Build history of the part. All positions in model axes, mm. A direction names the side the tool comes from. Round coordinates to 2 decimals unless told otherwise and drop trailing zeros. Write each loop counter-clockwise with the first axis right and the second up, starting at its lowest first coordinate (ties: lowest second). Pieces come first, ordered by that corner, then holes. Notation, with made-up numbers: M 47,87 L 57,87 A24 cw 57,115 Z; hole C 84,26 d9. An arc over 180 degrees is marked long. One line per item, written item: value. Start each with the question number.
```python
from build123d import *

# Parameters (mm, degrees)
F0_R     = 2.38125
F1_DEPTH = 3.175
F2_DEPTH = 4.7625
F3_T     = -1.5875
F4_R     = 3.175
F4_R_2   = 2.38125
F5_DEPTH = 1.5875


with BuildPart() as f1:
    # F0 (on Top) → F1 (new body)
    with BuildSketch(Plane.XY):
        Polygon((0, 15.875), (-7.9375, 15.875), (-7.9375, -15.875), (7.9375, -15.875), align=None)
        with Locations((-3.96875, -11.90625)):
            Circle(F0_R, mode=Mode.SUBTRACT)
        with Locations((-3.96875, -3.96875)):
            Circle(F0_R, mode=Mode.SUBTRACT)
        with Locations((-3.96875, 3.96875)):
            Circle(F0_R, mode=Mode.SUBTRACT)
        with Locations((-3.96875, 11.90625)):
            Circle(F0_R, mode=Mode.SUBTRACT)
    extrude(amount=F1_DEPTH)

    # F0 (on Top) → F2 (join)
    with BuildSketch(Plane.XY):
        with Locations((-3.96875, 11.90625)):
            Circle(F0_R)
        with Locations((-3.96875, 3.96875)):
            Circle(F0_R)
        with Locations((-3.96875, -3.96875)):
            Circle(F0_R)
        with Locations((-3.96875, -11.90625)):
            Circle(F0_R)
    extrude(amount=F2_DEPTH)

    # F3
    f3_openings = [f1.faces().sort_by_distance(p)[0] for p in [
        (-1.763889, -1.763889, 0),
    ]]
    offset(amount=F3_T, openings=f3_openings, kind=Kind.INTERSECTION)

    # F2_face (on face) + F4 (on face) → F5 (join)
    with BuildSketch(Plane(origin=(-1.7638745265, -1.3908157983, 0), x_dir=(1, 0, 0), z_dir=(0, 0, -1))):
        Polygon((-6.1736254735, -17.2658157983), (1.7638745265, -17.2658157983), (9.7013745265, 14.4841842017), (-6.1736254735, 14.4841842017), align=None)
        Polygon((0.5243919814, -15.6783157983), (-4.5861254735, -15.6783157983), (-4.5861254735, 12.8966842017), (7.6681419814, 12.8966842017), align=None, mode=Mode.SUBTRACT)
    with BuildSketch(Plane(origin=(0, 0, 1.5875), x_dir=(1, 0, 0), z_dir=(0, 0, -1))):
        with BuildLine():
            Line((0.8992491716, -5.7325731328), (1.0932302062, -4.9566489946))
            ThreePointArc((1.0932302062, -4.9566489946), (-3.080202438, -7.1674493905), (-0.4381385265, -11.0821239253))
            Line((-0.4381385265, -11.0821239253), (-0.244157492, -10.3061997871))
            ThreePointArc((-0.244157492, -10.3061997871), (-2.3101518285, -7.3599620429), (0.8992491716, -5.7325731328))
        make_face()
        with BuildLine():
            ThreePointArc((2.7353766172, 1.6119366495), (-3.080202438, 0.7700506095), (1.6550091801, -2.7095330988))
            Line((1.6550091801, -2.7095330988), (2.0152745824, -1.2684714896))
            ThreePointArc((2.0152745824, -1.2684714896), (-2.3101518285, 0.5775379571), (2.3751112149, 0.1708750402))
            Line((2.3751112149, 0.1708750402), (2.7353766172, 1.6119366495))
        make_face()
        with Locations((0, 7.9375)):
            Circle(F4_R)
        with Locations((0, 7.9375)):
            Circle(F4_R_2, mode=Mode.SUBTRACT)
    extrude(amount=F5_DEPTH)


solid = f1.part
```
Item 1: Two-plate mould, pull along X, no slides. Class faces 4 (the flat face through (-4, 12, 4.762)), 5 (the cylindrical face through (-1.697, 4.684, 3.958)), 6 (the cylindrical face through (-2.33, -0.49, 0.8)), 7 (the cylindrical face through (-3.061, 7.095, 0.805)): pulls with the +X half, pulls with the -X half, needs draft (parallel to the pull), parting line crosses it, or undercut.
Item 2: Cut at C-C, the plane z = 2.25. Write the cut outline in (x, y) (1 decimal), plus the area to 3 significant figures.
Item 3: Drop flat-ended pins along their axis: pin 1 (4.5 mm diameter, centred on x = 0, y = -7.94, fed in from +Z) (3 decimals); pin 2 (3 mm diameter, centred on x = -0.5, y = -9, fed in from -Z); pin 3 (2 mm diameter, centred on x = -3.97, y = -11.91, fed in from -Z). Give the stop position or say it passes through.
Item 4: Drill centre lines: line 1 (Y direction, x = -3.5, z = -0.25) (1 decimal); line 2 (Z direction, x = -0.25, y = -5) (3 decimals); line 3 (X direction, y = 12, z = 4). Where is each one in solid material? Low to high.
Item 5: Cut at A-A, the plane z = 0.5. Count the separate pieces of the cut face and the enclosed holes in it, plus the area to 3 significant figures.
Item 6: Which spindle directions (+Z, -Z, +X, -X, +Y, -Y) get a long thin tool onto all of the face, cutting with end or side? Do faces 1 (the flat face through (0, -3, 3.175)), 2 (the flat face through (-4, -12, 3.175)), 3 (the flat face through (-4, -12, 4.762)). Say none if no direction does.
Computed values:
1. face 4: needs draft
1. face 5: parting line crosses it
1. face 6: undercut
1. face 7: undercut
2. outline: M -7.9,-15.9 L 7.9,-15.9 L 0,15.9 L -7.9,15.9 Z; hole C -4,-11.9 d1.6; hole C -4,-4 d1.6; hole C -4,4 d1.6; hole C -4,11.9 d1.6
2. area: 370 mm2
3. pin 1: stops at z = 3.175
3. pin 2: stops at z = 0
3. pin 3: stops at z = 1.59
4. line 1: y = -15.9 to -14.3, 14.3 to 15.9
4. line 2: z = 0 to 3.175
4. line 3: x = -6.35 to -1.59
5. separate pieces: 2
5. enclosed holes: 4
5. area: 162 mm2
6. face 1: +Z
6. face 2: -Z
6. face 3: +Z, +X, -X, +Y, -Y
